Build history of the part. All positions in model axes, mm. Face numbers are marked on the shaded views. Give positions to 0.01 mm unless a question says otherwise; leave off trailing zeros. Order: outer loops, then holes, each group sorted by start corner. A loop starts at its lowest first (then second) coordinate and runs counter-clockwise, first axis right, second up. Notation, with made-up numbers: M -8,-11 L 39,-11 A24 cw 39,2 Z; hole C -37.75,-4.5 d2. An arc over 180 degrees is marked long. One line per item, written item: value.
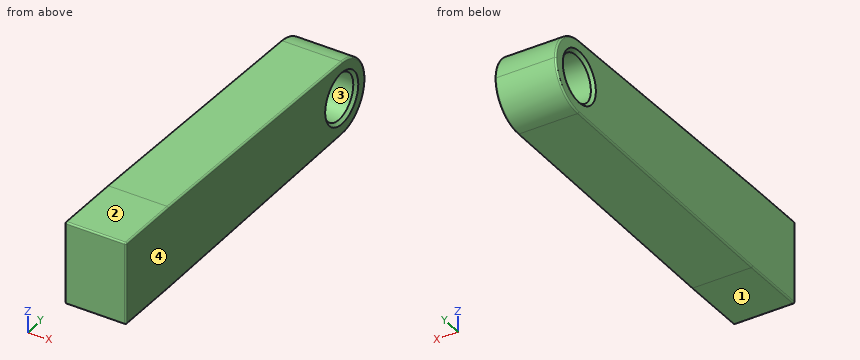
from build123d import *

# Parameters (mm, degrees)
F0_W     = 109.173186
F0_H     = 135
F0_R     = 37.5
F1_DEPTH = 100
F2_R     = 2.5
F3_SIZE  = 5


with BuildPart() as f1:
    # F0 (on Right) → F1 (new body)
    with BuildSketch(Plane.YZ):
        Rectangle(F0_W, F0_H)
        with BuildLine():
            Line((501.009012, 59.991515), (54.586593, 67.5))
            Line((54.586593, 67.5), (54.586593, -67.5))
            Line((54.586593, -67.5), (501.009012, -59.991515))
            ThreePointArc((501.009012, -59.991515), (440, 0), (501.009012, 59.991515))
        make_face()
        with BuildLine():
            ThreePointArc((560, 0), (542.781659, 42.068155), (501.009012, 59.991515))
            ThreePointArc((501.009012, 59.991515), (440, 0), (501.009012, -59.991515))
            ThreePointArc((501.009012, -59.991515), (542.781659, -42.068155), (560, 0))
        make_face()
        with Locations((500, 0)):
            Circle(F0_R, mode=Mode.SUBTRACT)
    extrude(amount=F1_DEPTH)

    # F2
    f2_edges = [f1.edges().sort_by_distance(p)[0] for p in [
        (100, 277.797802, 63.745758),
        (100, 277.797802, -63.745758),
        (100, 0, -67.5),
        (100, -54.586593, 0),
        (100, 0, 67.5),
        (100, 560, 0),
        (0, 277.797802, 63.745758),
        (0, 560, 0),
        (0, 277.797802, -63.745758),
        (0, 0, -67.5),
        (0, -54.586593, 0),
        (0, 0, 67.5),
        (50, -54.586593, -67.5),
        (50, -54.586593, 67.5),
    ]]
    fillet(f2_edges, radius=F2_R)

    # F3
    f3_edges = [f1.edges().sort_by_distance(p)[0] for p in [
        (100, 462.5, 0),
        (0, 462.5, 0),
    ]]
    chamfer(f3_edges, length=F3_SIZE)


solid = f1.part
1) Saw through at A-A, the plane x = 33. Write the cut outline in (y, z), then the cut area to 3 significant figures.
Check values:
outline: M -54.59,-65 A2.5 ccw -52.09,-67.5 L 54.59,-67.5 L 501.01,-59.99 A60 ccw 501.01,59.99 L 54.59,67.5 L -52.09,67.5 A2.5 ccw -54.59,65 Z; hole C 500,0 d75
area: 72,800 mm^2
2) Drill centre lines: probe 1 along Z at (x, y) = (33, 500); probe 2 along Z at (x, y) = (78.5, 513.5); probe 3 along Y at (x, z) = (94, -4.5). Where is each one in solid material? Low to high. Write a range as from..to.
Check values:
probe 1: -60.01..-37.5, 37.5..60.01
probe 2: -58.46..-34.99, 34.99..58.46
probe 3: -54.59..462.77, 537.23..559.83
3) Mould opens along Z. For the marked faces 1, 2, 3 and 4 say: released by +Z, released by -Z, zero draft, split by the parting line, or undercut.
Check values:
face 1: released by -Z
face 2: released by +Z
face 3: undercut
face 4: zero draft
4) Pin check, flat tips, straight feed: pin 1 (5 mm diameter, centred on x = 13, y = 428, fed in from +Z); pin 2 (3 mm diameter, centred on x = 69.5, y = 338.5, fed in from +Z); pin 3 (4 mm diameter, centred on x = 40.5, z = -8.5, fed in from +Y). Stop position of each tip, or through.
Check values:
pin 1: z = 61.26
pin 2: z = 62.75
pin 3: y = 559.65
